Part model, mm, in its own coordinate system. Face numbers are marked on the shaded views. A direction names the side the tool comes from. Round coordinates to 2 decimals unless told otherwise and drop trailing zeros. Loops run counter-clockwise (first coordinate to the right, second up) from the corner with the lowest first, then second, coordinate; pieces in that order, holes last.
(1) Tool access for the marked faces 5 and 6: list every direction of +Z, -Z, +X, -X, +Y, -Y with a clear straight run to the whole face (end or side of a thin tool).
(2) Cut at A-A on z = -32.5. List the corners of the cut face in (x, y), then the cut area to 3 significant figures.
(3) Flat gauge pins, fed straight in: pin 1 (1 mm diameter, centred on y = -1.5, z = -32, fed in from -X); pin 2 (3 mm diameter, centred on y = 1, z = -17.5, fed in from +X); pin 3 (1.5 mm diameter, centred on y = -1.5, z = -31.5, fed in from +X); pin 4 (1.5 mm diameter, centred on x = 0.5, z = -22, fed in from -Y). Where does each tip first touch, or does it go through?
(4) Probe probe 1 along Y at (x, z) = (0, -14.85); probe 2 along Z at (x, y) = (-0.5, -0.5); probe 3 along Z at (x, y) = (0.5, -1.5). List the from-to ranges inside material, lowest first.
(5) Mould opens along Y. For the marked faces 1, 2, 3 and 4 say: +Y half, -Y half, draft (parallel to the pull), parting line (faces both ways), or undercut.
Autodesk Inventor part; units mm, degrees
ref_plane "MSC_PF1" through (0, 0, 0) normal (0, 1, 0) x (-1, 0, 0)
ref_plane "MSC_PT1" through (0, 0, -16.7994) normal (0, 0, -1) x (-1, 0, 0)
ref_plane "YZ Plane" through (0, 0, 0) normal (1, 0, 0) x (0, 1, 0)
sketch "Skizze2" plane through (0, 0, 0) normal (0, 1, 0) x (-1, 0, 0)
  line L0 (0, -16.7994) -> (0, -36.7994)
  line L1 (0, -36.7994) -> (1.25, -36.7994)
  line L2 (1.5, -36.5494) -> (1.5, -24.7994)
  line L3 (1.5, -24.7994) -> (1.3, -24.453)
  line L4 (1.3, -24.453) -> (1.3, -16.7994)
  line L5 (1.3, -16.7994) -> (0, -16.7994)
  line L6 (1.25, -36.7994) -> (1.5, -36.5494)
  line L7 (1.5, -36.7994) -> (1.5, -37.153)
  line L8 (0, -41.2237) -> (0, -12.7287)
  dimension "Ds" = 2.6
  dimension "NND" = 3
  dimension "b" = 12
  dimension "d3" = 30
  dimension "d5" = 45
  dimension "PTC" = 0.5
  dimension "NLG" = 20
revolve "Drehung1" add sketch "Skizze2" angle 360 about axis through (0, 0, -16.7994) along (0, 0, -1)
sketch "Skizze3" plane through (0, 0, -16.7994) normal (0, 0, 1) x (1, 0, 0)
  circle A0 centre (0, 0) radius 1.3
  line L0 (0, 2.75) -> (1.5877, 2.75)
  line L1 (1.5877, 2.75) -> (3.1754, 0)
  line L2 (3.1754, 0) -> (0, 0)
  line L3 (0, 0) -> (0, 2.75)
  line L4 (0, 2.75) -> (-1.5877, 2.75)
  line L5 (-1.5877, 2.75) -> (-3.1754, 0)
  line L6 (0, -2.75) -> (1.5877, -2.75)
  line L7 (1.5877, -2.75) -> (3.1754, 0)
  line L8 (-1.5877, -2.75) -> (-3.1754, 0)
  line L9 (0, -2.75) -> (-1.5877, -2.75)
  dimension "d9" = 60
  dimension "ParS" = 5.5
  dimension "msp_d11" = 5.5
extrude "Extrusion1" add sketch "Skizze3" along normal blind 2
sketch "Skizze4" plane through (0, 0, 0) normal (0, 1, 0) x (-1, 0, 0)
  line L0 (-2.75, -14.7994) -> (-3.1754, -14.7994)
  line L1 (-3.1754, -14.7994) -> (-3.1754, -15.045)
  line L2 (-3.1754, -15.045) -> (-2.75, -14.7994)
  line L3 (0, -25.6442) -> (0, 36.2691)
  line L4 (0, 27.4244) -> (0, 27.1787)
  line L5 (-3.1754, -16.7994) -> (-3.1754, -14.7994)
  line L6 (-1.5877, -14.7994) -> (-3.1754, -14.7994)
  dimension "d14" = 30
  dimension "msp_d15" = 5.5
revolve "Drehung2" cut sketch "Skizze4" angle 360 about axis through (0, 0, 27.4244) along (0, 0, -1)
sketch "Sketch5" plane through (0, 0, -14.7994) normal (0, 0, 1) x (1, 0, 0)
  arc A0 (2.3816, 1.375) -> (0, 2.75) centre (0, 0) ccw
  circle A1 centre (0, 0) radius 2.0625
  dimension "d27" = 4.125
extrude "Extrusion2" cut sketch "Sketch5" against normal blind 0.4
thread "Gewinde1"
ref_plane "MSC_PF1" through (0, 0, 0) normal (0, 1, 0) x (-1, 0, 0)
ref_plane "MSC_PT1" through (0, 0, -16.7994) normal (0, 0, -1) x (-1, 0, 0)
fillet "Fillet1" radius 0.1 1 edges at (1.3, 0, -16.7994)
equation "\"msp_d11\" = ParS"
equation "\"d27\" = 0.75 * ParS"
equation "\"d28\" = 0.2 * ParK"
equation "\"d30\" = r"
equation "\"msp_d17\" = b"
equation "\"msp_d15\" = ParS"
equation "\"r\" = 0.1"
equation "\"THREADDIA\" = NND"
properties part number "DIN EN ISO 4015 - M3x20" material "Edelstahl, 440C"
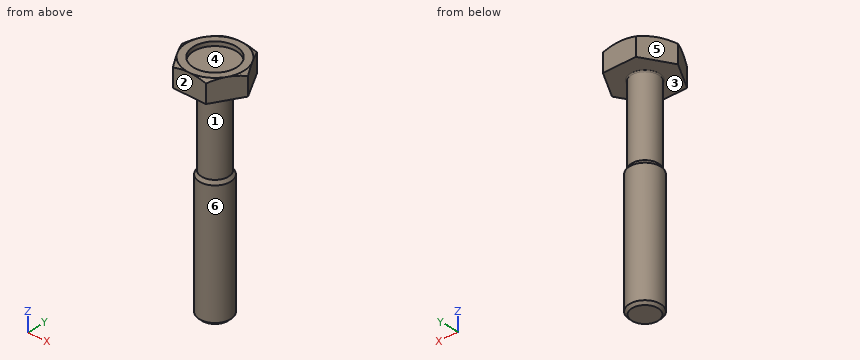
Final values:
1. face 5: +Z, -Z, -X, +Y
1. face 6: -Z
2. outline: circle Ø3 at (0, 0)
2. area: 7.07 mm2
3. pin 1: stops at x = -1.12
3. pin 2: stops at x = 3.18
3. pin 3: stops at x = 1.3
3. pin 4: stops at y = -1.3
4. probe 1: y = -2.75 to -2.06, 2.06 to 2.75
4. probe 2: z = -36.8 to -15.2
4. probe 3: z = -16.8 to -15.2
5. face 1: parting line
5. face 2: -Y half
5. face 3: draft
5. face 4: undercut
